Study the drawing (mm; zero at the part's minimum x, y, z) and answer. A direction names the side the tool comes from. Coordinates: 2 decimals unless noted, no trailing zeros. Order: outer loops, then holes, each group sorted by start corner. A loop starts at its lowest first (then second) coordinate and runs counter-clockwise, first axis right, second up. Notation, with made-up numbers: (76, 28.25) -> (126, 28.25) arc R31 cw to (126, 60.25) -> close; hole circle Ø11 at (56.25, -26.5). An arc over 180 degrees is marked (long way). One line per question, with ' | ' between items.
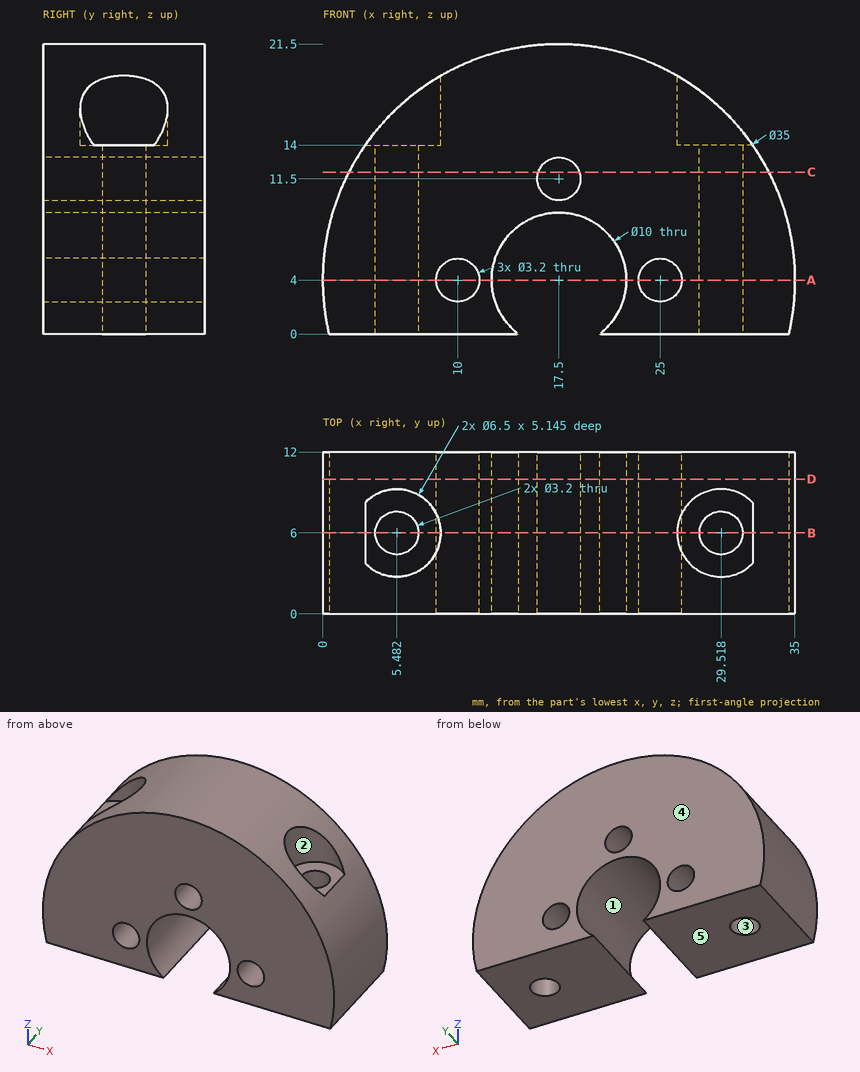
Item 1: For the marked faces 1 and 2, determine the directions among +Z, -Z, +X, -X, +Y, -Y from which every point of the face is accessible in a straight line to the end or side of a thin tool.
Computed values:
face 1: +Y, -Y | face 2: +Z
Item 2: Find the intervals of material crossed by L1, parallel to X at y = 8.5, z = 4; L2, parallel to X at y = 3, z = 3.5 (1 decimal); L3, parallel to X at y = 7.25, z = 13.75 (1 decimal), in increasing order.
Computed values:
L1: x = 0 to 8.4, 11.6 to 12.5, 22.5 to 23.4, 26.6 to 35 | L2: x = 0 to 8.5, 11.5 to 12.5, 22.5 to 23.5, 26.5 to 35 | L3: x = 3 to 4.5, 6.5 to 28.5, 30.5 to 32
Item 3: Determine the mould class of the marked faces 3, 4 and 5 for opening direction Y: pulls with the +Y half, pulls with the -Y half, needs draft (parallel to the pull), parting line crosses it, or undercut.
Computed values:
face 3: undercut | face 4: pulls with the +Y half | face 5: needs draft
Item 4: Section D-D, the plane y = 10 is taken. Give the vertices of the cut face in (x, z).
Computed values:
outline: (0.46, 0) -> (14.5, 0) arc R5 cw (long way) to (20.5, 0) -> (34.54, 0) arc R17.5 ccw (long way) to start; hole circle Ø3.2 at (10, 4); hole circle Ø3.2 at (17.5, 11.5); hole circle Ø3.2 at (25, 4)
Item 5: Section A-A, the plane z = 4 is taken. Give the vertices of the cut face in (x, y).
Computed values:
outline: (0, 0) -> (8.4, 0) -> (8.4, 12) -> (0, 12) -> close; (11.6, 0) -> (12.5, 0) -> (12.5, 12) -> (11.6, 12) -> close; (22.5, 0) -> (23.4, 0) -> (23.4, 12) -> (22.5, 12) -> close; (26.6, 0) -> (35, 0) -> (35, 12) -> (26.6, 12) -> close; hole circle Ø3.2 at (5.48, 6); hole circle Ø3.2 at (29.52, 6)
Item 6: Section C-C, the plane z = 12 is taken. Give the vertices of the cut face in (x, y) (1 decimal), plus the area to 3 significant figures.
Computed values:
outline: (1.9, 0) -> (16, 0) -> (16, 12) -> (1.9, 12) -> close; (19, 0) -> (33.1, 0) -> (33.1, 12) -> (19, 12) -> close; hole circle Ø3.2 at (5.5, 6); hole circle Ø3.2 at (29.5, 6) | area: 321 mm^2
Item 7: Each of these flat-tipped pins is pushed along its axis until it touches: pin 1 Ø5 at (y, z) = (10, 13.5) entering from +X; pin 2 Ø4 at (x, y) = (29.52, 6) entering from +Z; pin 3 Ø4.5 at (x, y) = (5, 7.5) entering from +Z (1 decimal); pin 4 Ø9 at (x, z) = (17.5, 4) entering from +Y. Where does it stop, or does it pass through?
Computed values:
pin 1: stops at x = 33.54 | pin 2: stops at z = 14 | pin 3: stops at z = 17.7 | pin 4: passes through
Item 8: Section B-B, the plane y = 6 is taken. Give the vertices of the cut face in (x, z) (1 decimal).
Computed values:
outline: (0.5, 0) -> (3.9, 0) -> (3.9, 14) -> (3.1, 14) arc R17.5 ccw to start; (7.1, 0) -> (14.5, 0) arc R5 cw (long way) to (20.5, 0) -> (27.9, 0) -> (27.9, 14) -> (26.3, 14) -> (26.3, 19.1) arc R17.5 ccw to (8.7, 19.1) -> (8.7, 14) -> (7.1, 14) -> close; (31.1, 0) -> (34.5, 0) arc R17.5 ccw to (31.9, 14) -> (31.1, 14) -> close; hole circle Ø3.2 at (10, 4); hole circle Ø3.2 at (17.5, 11.5); hole circle Ø3.2 at (25, 4)
